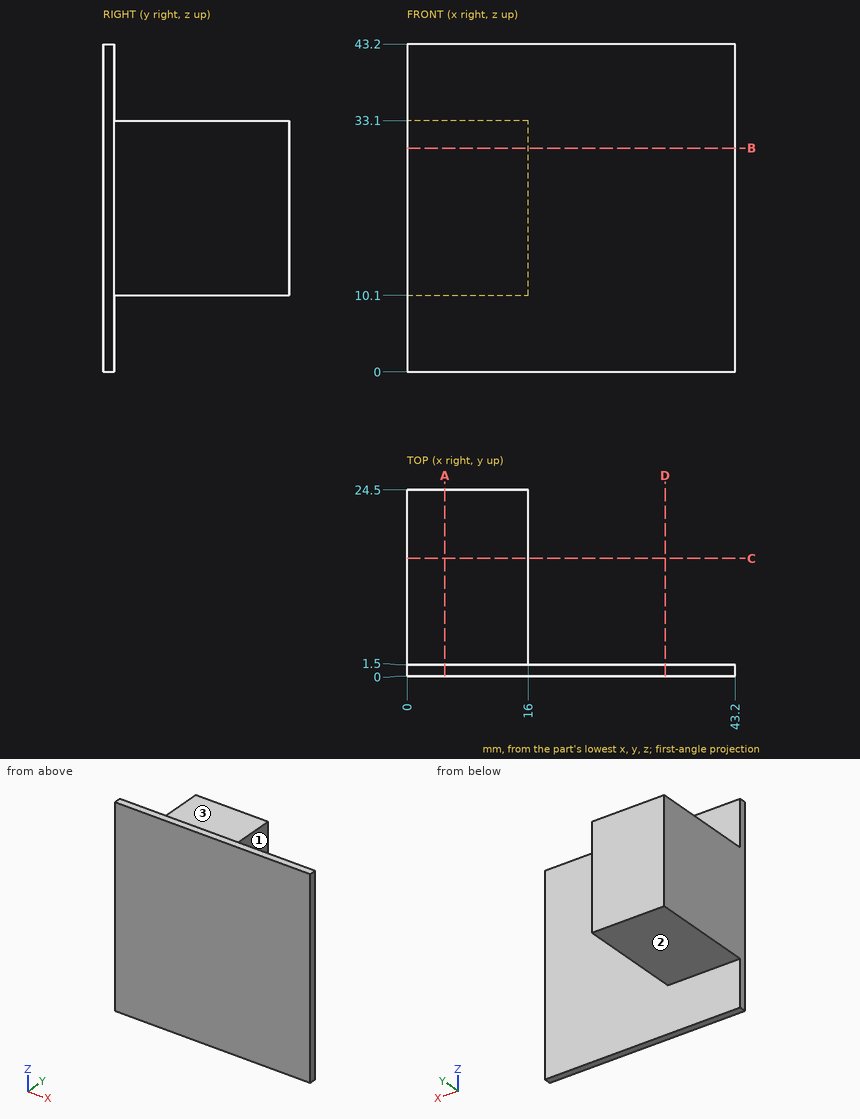
Design review of the part shown in the three views and the two pictorial views. Dimensions are in mm from the part's minimum x, y and z. A direction names the side the tool comes from. Give positions to 0.01 mm unless a question says otherwise; leave off trailing zeros. Write each loop counter-clockwise with the first axis right and the second up, starting at its lowest first coordinate (ties: lowest second). Pieces come first, ordered by that corner, then holes.
(1) Add section B-B (z = 29.5). Give the boundary of the cut face in (x, y), and give its area (3 significant figures).
Checked values:
outline: (0, 0) - (43.2, 0) - (43.2, 1.5) - (16, 1.5) - (16, 24.5) - (0, 24.5) - close
area: 433 mm2
(2) Add section C-C (y = 15.5). Give the boundary of the cut face in (x, z), and give its area (3 significant figures).
Checked values:
outline: (0, 10.1) - (16, 10.1) - (16, 33.1) - (0, 33.1) - close
area: 368 mm2
(3) Add section D-D (x = 34). Give the boundary of the cut face in (y, z), and give its area (3 significant figures).
Checked values:
outline: (0, 0) - (1.5, 0) - (1.5, 43.2) - (0, 43.2) - close
area: 64.8 mm2
(4) Clearance check with flat-ended pins moving along their axes: pin 1 Ø2 at (x, z) = (7.5, 21) entering from -Y; pin 2 Ø6 at (x, y) = (16.5, 16) entering from +Z; pin 3 Ø3 at (y, z) = (10.5, 25) entering from +X; pin 4 Ø2 at (x, y) = (24.5, 3.5) entering from +Z. State where each tip first meets the part, or that it passes through.
Checked values:
pin 1: stops at y = 0
pin 2: stops at z = 33.1
pin 3: stops at x = 16
pin 4: passes through
(5) Wall thickness on line 1 along Y through (x, z) = (31, 31); line 2 along Z through (x, y) = (14, 20.25); line 3 along X through (y, z) = (11.25, 21): over which ranges is each line inside the solid? List them lowest first.
Checked values:
line 1: y = 0 to 1.5
line 2: z = 10.1 to 33.1
line 3: x = 0 to 16
(6) Tool access review of the marked faces 1, 2 and 3: name each direction out of +Z, -Z, +X, -X, +Y, -Y from which nothing blocks a thin tool from reaching the whole face with its end or side.
Checked values:
face 1: +Z, -Z, +X, +Y
face 2: -Z, +X, -X, +Y
face 3: +Z, +X, -X, +Y
(7) Add section A-A (x = 5). Give the boundary of the cut face in (y, z).
Checked values:
outline: (0, 0) - (1.5, 0) - (1.5, 10.1) - (24.5, 10.1) - (24.5, 33.1) - (1.5, 33.1) - (1.5, 43.2) - (0, 43.2) - close
